Autodesk Inventor part; units mm, degrees
ref_plane "Arbeitsebene1" through (0, 0, 14) normal (0, 0, 1) x (1, 0, 0)
ref_plane "YZ Plane" through (0, 0, 0) normal (1, 0, 0) x (0, 1, 0)
ref_plane "XZ Plane" through (0, 0, 0) normal (0, 1, 0) x (-1, 0, 0)
sketch "Skizze1" plane through (0, 0, 0) normal (0, 0, 1) x (1, 0, 0)
  line L0 (-10, -30) -> (10, -30)
  line L1 (10, -30) -> (10, 30)
  line L2 (10, 30) -> (-10, 30)
  line L3 (-10, 30) -> (-10, -30)
extrude "Extrusion1" add sketch "Skizze1" along normal blind 14
sketch "Skizze2" plane through (0, 0, 0) normal (0, 0, 1) x (1, 0, 0)
  circle A0 centre (0, -22) radius 3.9
extrude "Extrusion2" cut sketch "Skizze2" along normal blind 10
sketch "Skizze3" plane through (0, 0, 0) normal (0, 0, 1) x (1, 0, 0)
  circle A0 centre (0, 22) radius 3.9
extrude "Extrusion3" cut sketch "Skizze3" along normal blind 10
ref_plane "Arbeitsebene1" through (0, 0, 14) normal (0, 0, 1) x (1, 0, 0)
sketch "Skizze4" plane through (0, 0, 14) normal (0, 0, 1) x (1, 0, 0)
  circle A0 centre (0, 0) radius 5.25
extrude "Extrusion4" cut sketch "Skizze4" against normal blind 14.2
properties part number "Kopf_Bruecke"
Part model, mm, in its own coordinate system. A direction names the side the tool comes from. Coordinates: 2 decimals unless noted, no trailing zeros. Loops run counter-clockwise (first coordinate to the right, second up) from the corner with the lowest first, then second, coordinate; pieces in that order, holes last. Notation, with made-up numbers: M -18.75,19 L 37.25,19 A21 cw 37.25,30 Z; hole C 9.5,-6 d11. An arc over 180 degrees is marked long. Use a Markdown table: item, result. Add a question column.
Q1. Probe L1, parallel to Y at x = 0, z = 7.25; L2, parallel to Y at x = 1.5, z = 8.25; L3, parallel to Z at x = 2.5, y = -21. List the from-to ranges inside material, lowest first.
Q2. Cut at D-D (y = 22). Write the cut outline in (x, z), and give its area (3 significant figures).
Q3. Cut at A-A (y = 0). Write the cut outline in (x, z), and give its area (3 significant figures).
Q4. Cut at C-C (x = 0). Write the cut outline in (y, z).
Q5. Pin check, flat tip, straight feed: P1, Ø6, axis at x = 0, y = -21.5, coming from the -Z side. Stop position of the tip, or through.
Q6. Which spindle directions (+Z, -Z, +X, -X, +Y, -Y) get a long thin tool onto all of the face, cutting with end or side? Do faces 5 (the flat face through (-10, 0, 7)), 6 (the flat face through (0, 22, 10)). Say none if no direction does.
Q7. Cut at B-B (z = 4). Write the cut outline in (x, y).
Q8. Mould opens along Y. For faces 1 (the cylindrical face through (-0.845, -18.193, 4.93)), 2 (the flat face through (0, 7, 0)), 3 (the flat face through (0, 30, 7)), 4 (the flat face through (0, -30, 7)) say: +Y half, -Y half, draft (parallel to the pull), parting line (faces both ways), or undercut.
Worked out:
| question | item | result |
|---|---|---|
| 1 | L1 | y = -30 to -25.9, -18.1 to -5.25, 5.25 to 18.1, 25.9 to 30 |
| 1 | L2 | y = -30 to -25.6, -18.4 to -5.03, 5.03 to 18.4, 25.6 to 30 |
| 1 | L3 | z = 10 to 14 |
| 2 | outline | M -10,0 L -3.9,0 L -3.9,10 L 3.9,10 L 3.9,0 L 10,0 L 10,14 L -10,14 Z |
| 2 | area | 202 mm2 |
| 3 | outline | M -10,0 L -5.25,0 L -5.25,14 L -10,14 Z; M 5.25,0 L 10,0 L 10,14 L 5.25,14 Z |
| 3 | area | 133 mm2 |
| 4 | outline | M -30,0 L -25.9,0 L -25.9,10 L -18.1,10 L -18.1,0 L -5.25,0 L -5.25,14 L -30,14 Z; M 5.25,0 L 18.1,0 L 18.1,10 L 25.9,10 L 25.9,0 L 30,0 L 30,14 L 5.25,14 Z |
| 5 | P1 | stops at z = 10 |
| 6 | face 5 | +Z, -Z, -X, +Y, -Y |
| 6 | face 6 | -Z |
| 7 | outline | M -10,-30 L 10,-30 L 10,30 L -10,30 Z; hole C 0,0 d10.5; hole C 0,-22 d7.8; hole C 0,22 d7.8 |
| 8 | face 1 | undercut |
| 8 | face 2 | draft |
| 8 | face 3 | +Y half |
| 8 | face 4 | -Y half |
